from build123d import *

# Parameters (mm, degrees)
CYLINDER015_R     = 3.8
CYLINDER015_DEPTH = 3.2
CYLINDER014_R     = 18.3
CYLINDER014_DEPTH = 1.6
CYLINDER013_R     = 16.7
CYLINDER013_DEPTH = 3.2


with BuildPart() as zylinder015:
    # Cylinder015 → Cylinder015 (new body)
    with BuildSketch(Plane(origin=(130, 69.1, 0), x_dir=(1, 0, 0), z_dir=(0, 0, 1))):
        Circle(CYLINDER015_R)
    extrude(amount=CYLINDER015_DEPTH)


with BuildPart() as zylinder014:
    # Cylinder014 → Cylinder014 (new body)
    with BuildSketch(Plane(origin=(130, 69.1, 0), x_dir=(1, 0, 0), z_dir=(0, 0, 1))):
        Circle(CYLINDER014_R)
    extrude(amount=CYLINDER014_DEPTH)


with BuildPart() as ring:
    # Cylinder013 → Cylinder013 (new body)
    with BuildSketch(Plane(origin=(130, 69.1, 0), x_dir=(1, 0, 0), z_dir=(0, 0, 1))):
        Circle(CYLINDER013_R)
    extrude(amount=CYLINDER013_DEPTH)

    # Fusion010: union Zylinder014
    add(zylinder014.part)

    # Cut007: cut Zylinder015
    add(zylinder015.part, mode=Mode.SUBTRACT)


solid = ring.part
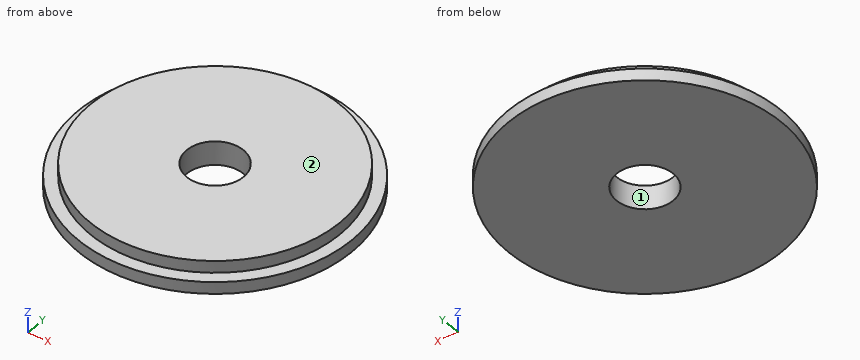
Read the model definition and answer for the solid it produces. Units are mm, in the model's axes. Face numbers are marked on the shaded views. Round coordinates to 2 decimals unless told otherwise and drop trailing zeros. Write each loop counter-clockwise with the first axis right and the second up, starting at its lowest first coordinate (ties: lowest second). Pieces come first, ordered by that corner, then holes.
Q1. Find section A-A on x = 130. Determine the outline of the cut face in (y, z).
Values:
outline: (50.8, 0) - (65.3, 0) - (65.3, 3.2) - (52.4, 3.2) - (52.4, 1.6) - (50.8, 1.6) - close; (72.9, 0) - (87.4, 0) - (87.4, 1.6) - (85.8, 1.6) - (85.8, 3.2) - (72.9, 3.2) - close
Q2. Find section C-C on x = 118.5. Determine the outline of the cut face in (y, z).
Values:
outline: (54.86, 0) - (83.34, 0) - (83.34, 1.6) - (81.21, 1.6) - (81.21, 3.2) - (56.99, 3.2) - (56.99, 1.6) - (54.86, 1.6) - close
Q3. A flat-ended cylindrical pin translates along its axis: P1, Ø4.5, axis at x = 130, y = 69.1, coming from the -Z side. Find the tip coordinate at first contact, or state that the pin passes through.
Values:
P1: passes through
Q4. Straight lines are drawn through the part: line 1 (Y direction, x = 130, z = 1.25); line 2 (Y direction, x = 130, z = 2.45); line 3 (X direction, y = 71.5, z = 3.1). For each, find the intervals that lie inside material, in ascending order.
Values:
line 1: y = 50.8 to 65.3, 72.9 to 87.4
line 2: y = 52.4 to 65.3, 72.9 to 85.8
line 3: x = 113.47 to 127.05, 132.95 to 146.53
Q5. Find section B-B on y = 69.1. Determine the outline of the cut face in (x, z).
Values:
outline: (111.7, 0) - (126.2, 0) - (126.2, 3.2) - (113.3, 3.2) - (113.3, 1.6) - (111.7, 1.6) - close; (133.8, 0) - (148.3, 0) - (148.3, 1.6) - (146.7, 1.6) - (146.7, 3.2) - (133.8, 3.2) - close
Q6. Find section D-D on z = 0.8. Determine the outline of the cut face in (x, y), and give its area (3 significant figures).
Values:
outline: circle Ø36.6 at (130, 69.1); hole circle Ø7.6 at (130, 69.1)
area: 1,010 mm2
Q7. The mould has two halves that part along Y. Classify the marked faces 1 and 2: released by +Y, released by -Y, zero draft, split by the parting line, or undercut.
Values:
face 1: undercut
face 2: zero draft
